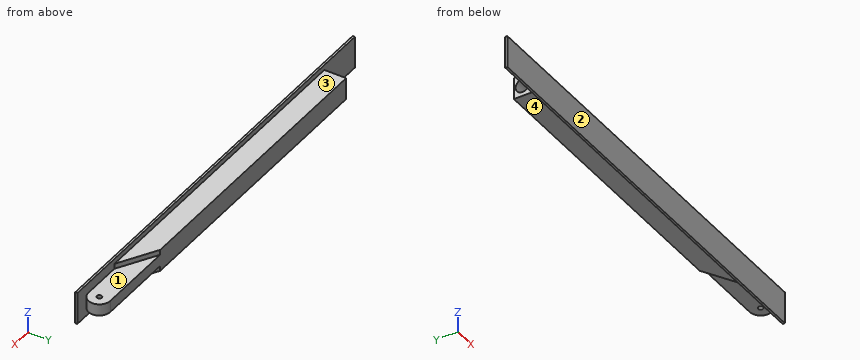
```python
from build123d import *

# Parameters (mm, degrees)
BOSS_EXTRUDE1_DEPTH      = 15
H_0_266_DIAMETER_HOLE1_D = 6.7564
SKETCH5_W                = 40
SKETCH5_H                = 16
SKETCH5_H_2              = 20.916111238
CUT_EXTRUDE1_DEPTH       = 243.332416321
SKETCH6_W                = 429.036778435
SKETCH6_H                = 127.431795429
CUT_EXTRUDE2_DEPTH       = 243.332416321
SKETCH10_W               = 30
SKETCH10_H               = 30
BOSS_EXTRUDE3_DEPTH      = 500
SKETCH11_R               = 9.525
CUT_EXTRUDE4_DEPTH       = 400
SKETCH13_W               = 600
SKETCH13_H               = 44.158972604
BOSS_EXTRUDE4_DEPTH      = 3
SKETCH14_W               = 111.034909532
SKETCH14_H               = 112.185530356
CUT_EXTRUDE5_DEPTH       = 30
CHAMFER1_SIZE            = 100
CHAMFER1_SIZE_2          = 57.735026919


with BuildPart() as part:
    # Sketch1 → Boss-Extrude1 (new, symmetric)
    with BuildSketch(Plane.XY):
        with BuildLine():
            Line((-225, 15), (225, 15))
            ThreePointArc((225, 15), (240, 0), (225, -15))
            Line((225, -15), (-225, -15))
            ThreePointArc((-225, -15), (-240, 0), (-225, 15))
        make_face()
    extrude(amount=BOSS_EXTRUDE1_DEPTH, both=True)

    # H (0.266) Diameter Hole1 (through all)
    with Locations(Plane.XY.offset(15)):
        with Locations((-225, 0), (225, 0)):
            Hole(H_0_266_DIAMETER_HOLE1_D / 2)

    # Sketch5 → Cut-Extrude1 (cut, through all)
    with BuildSketch(Plane(origin=(0, 15, 0), x_dir=(1, 0, 0), z_dir=(0, 1, 0))):
        with Locations((-237, 0)):
            Rectangle(SKETCH5_W, SKETCH5_H)
        with Locations((237, 18.458055619)):
            Rectangle(SKETCH5_W, SKETCH5_H_2)
        with Locations((237, -18.458055619)):
            Rectangle(SKETCH5_W, SKETCH5_H_2)
    extrude(amount=-CUT_EXTRUDE1_DEPTH, mode=Mode.SUBTRACT)

    # Sketch6 → Cut-Extrude2 (cut, through all)
    with BuildSketch(Plane(origin=(0, 15, 0), x_dir=(1, 0, 0), z_dir=(0, 1, 0))):
        with Locations((-47.518389218, -4.674139215)):
            Rectangle(SKETCH6_W, SKETCH6_H)
    extrude(amount=-CUT_EXTRUDE2_DEPTH, mode=Mode.SUBTRACT)

    # Sketch10 → Boss-Extrude3 (add)
    with BuildSketch(Plane.ZY.offset(-167)):
        Rectangle(SKETCH10_W, SKETCH10_H)
    extrude(amount=BOSS_EXTRUDE3_DEPTH)

    # Sketch11 → Cut-Extrude4 (cut)
    with BuildSketch(Plane.ZY.offset(333)):
        with Locations((0, 3)):
            Circle(SKETCH11_R)
    extrude(amount=-CUT_EXTRUDE4_DEPTH, mode=Mode.SUBTRACT)

    # Sketch13 → Boss-Extrude4 (add)
    with BuildSketch(Plane(origin=(0, -15, 0), x_dir=(-1, 0, 0), z_dir=(0, -1, 0))):
        with Locations((51, 0)):
            Rectangle(SKETCH13_W, SKETCH13_H)
    extrude(amount=BOSS_EXTRUDE4_DEPTH)

    # Sketch14 → Cut-Extrude5 (cut)
    with BuildSketch(Plane(origin=(0, 15, 0), x_dir=(1, 0, 0), z_dir=(0, 1, 0))):
        with Locations((-340.517454766, -2.301241648)):
            Rectangle(SKETCH14_W, SKETCH14_H)
    extrude(amount=-CUT_EXTRUDE5_DEPTH, mode=Mode.SUBTRACT)

    # Chamfer1
    # the kernel refuses this chamfer: 100, 57.735026919 mm, written as the material it takes off along each edge
    with BuildSketch(Plane(origin=(217, 15, 250.708575465), x_dir=(-0.9998132206222079, 0.01932676561270057, 2.717178209496515e-15), z_dir=(0, 0, -1))) as chamfer1_piece_1_section:
        Polygon((CHAMFER1_SIZE * 0.999813220622, -CHAMFER1_SIZE * 0.0193267656127), (-CHAMFER1_SIZE_2 * 0.0193267656127, -CHAMFER1_SIZE_2 * 0.999813220622), (0, 0), align=None)
    chamfer1_piece_1 = extrude(amount=524.417150929, mode=Mode.PRIVATE)
    chamfer1_piece_1 = split(chamfer1_piece_1, bisect_by=Plane(origin=(178.470505911, -15, 11.5), z_dir=(0, 1, 0)), keep=Keep.TOP, mode=Mode.PRIVATE)
    chamfer1_piece_1 = split(chamfer1_piece_1, bisect_by=Plane(origin=(178.470505911, 1.75500065, 8), z_dir=(0, 0, 1)), keep=Keep.TOP, mode=Mode.PRIVATE)
    add(chamfer1_piece_1, mode=Mode.SUBTRACT)
    with BuildSketch(Plane(origin=(217, 15, -8), x_dir=(-0.9998132206222079, 0.019326765612700587, 2.717178209496515e-15), z_dir=(0, 0, -1))) as chamfer1_piece_2_section:
        Polygon((CHAMFER1_SIZE * 0.999813220622, -CHAMFER1_SIZE * 0.0193267656127), (-CHAMFER1_SIZE_2 * 0.0193267656127, -CHAMFER1_SIZE_2 * 0.999813220622), (0, 0), align=None)
    chamfer1_piece_2 = extrude(amount=265.708575465, mode=Mode.PRIVATE)
    chamfer1_piece_2 = split(chamfer1_piece_2, bisect_by=Plane(origin=(178.470505911, -15, -11.5), z_dir=(0, 1, 0)), keep=Keep.TOP, mode=Mode.PRIVATE)
    add(chamfer1_piece_2, mode=Mode.SUBTRACT)
    with BuildSketch(Plane(origin=(217, 15, -250.708575465), x_dir=(0.057893862402671484, -0.9983227437537925, 0), z_dir=(0, 0, 1))) as chamfer1_piece_3_section:
        Polygon((CHAMFER1_SIZE_2 * 0.998322743753, -CHAMFER1_SIZE_2 * 0.0578938624026), (-CHAMFER1_SIZE * 0.0578938624027, -CHAMFER1_SIZE * 0.998322743754), (0, 0), align=None)
    chamfer1_piece_3 = extrude(amount=524.417150929, mode=Mode.PRIVATE)
    chamfer1_piece_3 = split(chamfer1_piece_3, bisect_by=Plane(origin=(178.470505911, -15, -11.5), z_dir=(0, 1, 0)), keep=Keep.TOP, mode=Mode.PRIVATE)
    chamfer1_piece_3 = split(chamfer1_piece_3, bisect_by=Plane(origin=(178.470505911, 1.75500065, -8), z_dir=(0, 0, -1)), keep=Keep.TOP, mode=Mode.PRIVATE)
    add(chamfer1_piece_3, mode=Mode.SUBTRACT)
    with BuildSketch(Plane(origin=(217, 15, 8), x_dir=(0.05789386240267099, -0.9983227437537925, 0), z_dir=(0, 0, 1))) as chamfer1_piece_4_section:
        Polygon((CHAMFER1_SIZE_2 * 0.998322743753, -CHAMFER1_SIZE_2 * 0.0578938624026), (-CHAMFER1_SIZE * 0.0578938624027, -CHAMFER1_SIZE * 0.998322743754), (0, 0), align=None)
    chamfer1_piece_4 = extrude(amount=265.708575465, mode=Mode.PRIVATE)
    chamfer1_piece_4 = split(chamfer1_piece_4, bisect_by=Plane(origin=(178.470505911, -15, 11.5), z_dir=(0, 1, 0)), keep=Keep.TOP, mode=Mode.PRIVATE)
    add(chamfer1_piece_4, mode=Mode.SUBTRACT)


solid = part.part
```
Input: part model. Units: mm. Frame: model coordinates. Face numbers are marked on the shaded views. A direction names the side the tool comes from. Give positions to 0.01 mm unless a question says otherwise; leave off trailing zeros. Loops run counter-clockwise (first coordinate to the right, second up) from the corner with the lowest first, then second, coordinate; pieces in that order, holes last. Notation, with made-up numbers: M -21,81 L -5,81 A20 ccw -5,93 Z; hole C 26,-8 d11. An arc over 180 degrees is marked long. Answer as CSV lines item,"result". Start each with the question number.
1. Section A-A on x = -186.5. Return loops of the section in (y, z) (3 decimals), plus the area to 3 significant figures.
2. Pin query (flat end, axial travel): P1, Ø15, axis at x = 193, y = 1.5, coming from the -Z side; P2, Ø9.5, axis at y = 4.5, z = -4, coming from the -X side; P3, Ø12, axis at x = -159.5, y = 4, coming from the -Z side; P4, Ø10, axis at y = -13.5, z = 8.5, coming from the -X side. Return the tip coordinate at first contact, or that it passes through.
3. Section C-C on x = -296.5. Return loops of the section in (y, z), plus the area to 3 significant figures.
4. Section B-B on z = 0. Return loops of the section in (x, y) (3 decimals).
5. Reachability of the marked faces 1, 2, 3 and 4 from +Z, -Z, +X, -X, +Y, -Y: full face, straight path, thin tool, end or side. Return the list, or none.
6. Line query: L1, parallel to Y at x = -16, z = 0 (3 decimals); L2, parallel to Z at x = 122.5, y = -13; L3, parallel to Z at x = -161.5, y = 11. Output: solid intervals per line, ascending.
Computed values:
1,outline,"M -18,-22.079 L -15,-22.079 L -15,-15 L 15,-15 L 15,15 L -15,15 L -15,22.079 L -18,22.079 Z; hole C 3,0 d19.05"
1,area,"747 mm²"
2,P1,"stops at z = -8"
2,P2,"stops at x = 67"
2,P3,"stops at z = -15"
2,P4,"stops at x = -351"
3,outline,"M -18,-22.08 L -15,-22.08 L -15,22.08 L -18,22.08 Z"
3,area,"132 mm²"
4,outline,"M -351,-18 L 249,-18 L 249,-15 L 225,-15 A15 ccw 225,15 L -285,15 L -285,12.525 L 67,12.525 L 67,-6.525 L -285,-6.525 L -285,-15 L -351,-15 Z; hole C 225,0 d6.756"
5,face 1,"+Z, +X, +Y"
5,face 2,"+Z, -Z, +X, -X, -Y"
5,face 3,"+Z, +X, -X, +Y"
5,face 4,"-Z, +X, -X, +Y"
6,L1,"y = -18 to -6.525, 12.525 to 15"
6,L2,"z = -15 to 15"
6,L3,"z = -15 to -5.17, 5.17 to 15"
